Check sheet for the modelled part. Datum: model origin and axes. Units: mm. Round coordinates to 2 decimals unless told otherwise and drop trailing zeros. Loops run counter-clockwise (first coordinate to the right, second up) from the corner with the lowest first, then second, coordinate; pieces in that order, holes last. Notation, with made-up numbers: (86, 56) -> (109, 56) arc R21 ccw to (109, 66) -> close; hole circle Ø7 at (55.25, 3). An arc over 180 degrees is marked (long way). One line per item, written item: value. Start each with the question number.
1. Material ranges on L1, parallel to Y at x = 1.5, z = 2; L2, parallel to Y at x = -14, z = 10; L3, parallel to X at y = 21, z = -5.5, recorded low to high.
2. Cross-section at C-C on x = 21. Record the cut outline in (y, z).
3. Cross-section at D-D on y = -10. Record the cut outline in (x, z).
4. Cross-section at A-A on x = 0. Record the cut outline in (y, z), then the cut area to 3 significant figures.
5. Release check for a two-part mould opening along Y. For faces 1 (the face through (35.05, 0.7, 32.94)), 2 (the face through (-1, -50, 0)), 3 (the face through (-0.511, -39.365, 4.776)) record: +Y half, -Y half, draft (parallel to the pull), parting line (faces both ways), or undercut.
6. Cross-section at B-B on z = 6. Record the cut outline in (x, y), then the cut area to 3 significant figures.
from build123d import *

# Parameters (mm, degrees)
F0_W     = 72.9447603226
F0_H     = 68.892262876
F1_DEPTH = 50
F3_R     = 5
F4_D     = 31.8
F6_D     = 32.14624


with BuildPart() as f1:
    # F0 (on Front) → F1 (new body, symmetric)
    with BuildSketch(Plane.XZ):
        Rectangle(F0_W, F0_H)
    extrude(amount=F1_DEPTH, both=True)

    # F3
    f3_edges = [f1.edges().sort_by_distance(p)[0] for p in [
        (36.47238, 0, 34.446131),
        (-36.47238, 0, 34.446131),
        (36.47238, 0, -34.446131),
        (-36.47238, 0, -34.446131),
    ]]
    fillet(f3_edges, radius=F3_R)

    # F4 (through all)
    with Locations(Plane.YZ.offset(36.4723801613)):
        with Locations((-24.1992101073, 0)):
            Hole(F4_D / 2)

    # F6 (through all)
    with Locations(Plane.XY.offset(34.446131438)):
        with Locations((0, 20.9348257631)):
            Hole(F6_D / 2)


solid = f1.part
Taken from the geometry:
1. L1: y = -50 to -39.97, -8.43 to 4.93, 36.94 to 50
1. L2: y = -50 to -36.56, -11.84 to 13.04, 28.83 to 50
1. L3: x = -36.47 to -16.07, 16.07 to 36.47
2. outline: (-50, -34.45) -> (50, -34.45) -> (50, 34.45) -> (-50, 34.45) -> close; hole circle Ø31.8 at (-24.2, 0)
3. outline: (-36.47, -29.45) arc R5 ccw to (-31.47, -34.45) -> (31.47, -34.45) arc R5 ccw to (36.47, -29.45) -> (36.47, -7.15) -> (-36.47, -7.15) -> close; (-36.47, 7.15) -> (36.47, 7.15) -> (36.47, 29.45) arc R5 ccw to (31.47, 34.45) -> (-31.47, 34.45) arc R5 ccw to (-36.47, 29.45) -> close
4. outline: (-50, -34.45) -> (4.86, -34.45) -> (4.86, 34.45) -> (-50, 34.45) -> close; (37.01, -34.45) -> (50, -34.45) -> (50, 34.45) -> (37.01, 34.45) -> close; hole circle Ø31.8 at (-24.2, 0)
4. area: 3,880 mm2
5. face 1: draft
5. face 2: -Y half
5. face 3: undercut
6. outline: (-36.47, -50) -> (36.47, -50) -> (36.47, -38.92) -> (-36.47, -38.92) -> close; (-36.47, -9.47) -> (36.47, -9.47) -> (36.47, 50) -> (-36.47, 50) -> close; hole circle Ø32.15 at (0, 20.93)
6. area: 4,330 mm2
